from build123d import *

# Parameters (mm, degrees)
F0_R     = 59.9289623747
F0_R_2   = 51.785848785
F1_DEPTH = 127
F3_DEPTH = 101.6
F4_DEPTH = 127
F5_R     = 34.7688744337
F6_DEPTH = 177.8


with BuildPart() as f1:
    # F0 (on Top) → F1 (new body)
    with BuildSketch(Plane.XY):
        Circle(F0_R)
        Circle(F0_R_2, mode=Mode.SUBTRACT)
        Circle(F0_R_2)
    extrude(amount=F1_DEPTH)

    # F3 (cut): a face of the model
    f3_faces = [f1.faces().sort_by_distance(p)[0] for p in [
        (0, 0, 127),
    ]]
    extrude(f3_faces, amount=-F3_DEPTH, mode=Mode.SUBTRACT)

    # F4 (add): a face of the model
    f4_faces = [f1.faces().sort_by_distance(p)[0] for p in [
        (0, 0, 25.4),
    ]]
    extrude(f4_faces, amount=F4_DEPTH)

    # F5 (on Top) → F6 (join)
    with BuildSketch(Plane.XY):
        Circle(F5_R)
    extrude(amount=F6_DEPTH)


solid = f1.part
For this review, take the finished solid that the model builds, in its own axes (mm). A direction names the side the tool comes from. Round coordinates to 2 decimals unless told otherwise and drop trailing zeros. Loops run counter-clockwise (first coordinate to the right, second up) from the corner with the lowest first, then second, coordinate; pieces in that order, holes last. Notation, with made-up numbers: (13, -36.5) - (62, -36.5) arc R5 cw to (62, -30.5) - close; hole circle Ø11 at (19, 57.5). An arc over 180 degrees is marked (long way). One line per item, written item: value. Start each with the question number.
Item 1: Clearance check with flat-ended pins moving along their axes: pin 1 Ø10 at (y, z) = (17, 158.5) entering from -X; pin 2 Ø4 at (x, z) = (-22, 48) entering from -Y; pin 3 Ø3 at (x, z) = (-42.5, 29.5) entering from -Y. State where each tip first meets the part, or that it passes through.
Item 2: Take a section at D-D (z = 60). Give the boundary of the cut face in (x, y), plus the area to 3 significant figures.
Item 3: Take a section at C-C (z = 167). Give the boundary of the cut face in (x, y).
Item 4: Take a section at A-A (x = 0). Give the boundary of the cut face in (y, z).
Item 5: For faces 1 (the flat face through (0, 0, 177.8)), 2 (the cylindrical face through (-4.526, 34.473, 164.922)), list the 3-axis set-ups (+Z, -Z, +X, -X, +Y, -Y) from which the entire face can be reached by the end or side of a thin tool; tool diameter is ignored.
Item 6: For L1, parallel to Z at x = 1, y = -48; L2, parallel to X at y = -51.5, z = 141.5; L3, parallel to Y at x = -6, z = 156.5, list the stretches that pass through material, from the lowest coordinate up.
Answer below:
1. pin 1: stops at x = -32.63
1. pin 2: stops at y = -56.49
1. pin 3: stops at y = -43.71
2. outline: circle Ø119.86 at (0, 0)
2. area: 11,300 mm2
3. outline: circle Ø69.54 at (0, 0)
4. outline: (-59.93, 0) - (59.93, 0) - (59.93, 152.4) - (34.77, 152.4) - (34.77, 177.8) - (-34.77, 177.8) - (-34.77, 152.4) - (-59.93, 152.4) - close
5. face 1: +Z, +X, -X, +Y, -Y
5. face 2: +Z
6. L1: z = 0 to 152.4
6. L2: x = -30.65 to 30.65
6. L3: y = -34.25 to 34.25
